Can you work these out from the model? Positions are in its coordinate system, mm. A direction names the side the tool comes from. Coordinates: 2 decimals unless noted, no trailing zeros. Loops run counter-clockwise (first coordinate to the right, second up) from the corner with the lowest first, then second, coordinate; pieces in that order, holes last.
```python
from build123d import *

# Parameters (mm, degrees)
SKETCH_2_R      = 5
EXTRUDE_1_DEPTH = 92
SKETCH_3_R      = 16
EXTRUDE_2_DEPTH = 25
SKETCH_4_R      = 16
SKETCH_4_R_2    = 11
EXTRUDE_3_DEPTH = 10
EXTRUDE_3_DRAFT = 5
FILLET_1_R      = 1


with BuildPart() as part:
    # 草图2 → 凸台-拉伸1 (new body)
    with BuildSketch(Plane(origin=(-136.095806698, 0, 0), x_dir=(0, 0, -1), z_dir=(1, 0, 0))):
        with Locations((-537.761833513, -181.314321461)):
            Circle(SKETCH_2_R)
    extrude(amount=-EXTRUDE_1_DEPTH)

    # 草图3 → 凸台-拉伸2 (add)
    with BuildSketch(Plane.ZY.offset(228.095806698)):
        with Locations((537.761833513, -181.314321461)):
            Circle(SKETCH_3_R)
    extrude(amount=EXTRUDE_2_DEPTH)


with BuildPart() as extrude_3_tool:
    # 草图4 → 凸台-拉伸3 (with draft: the straight prism first)
    with BuildSketch(Plane(origin=(-228.095806698, 0, 0), x_dir=(0, 0, -1), z_dir=(1, 0, 0))):
        with Locations((-537.761833513, -181.314321461)):
            Circle(SKETCH_4_R)
        with Locations((-537.761833513, -181.314321461)):
            Circle(SKETCH_4_R_2, mode=Mode.SUBTRACT)
    extrude(amount=EXTRUDE_3_DEPTH)
    # 凸台-拉伸3: the draft: its side faces are tilted about the plane it starts from
    extrude_3_sides = [extrude_3_tool.faces().sort_by_distance(p)[0] for p in [
        (-223.095806698, -181.314321461, 553.761833513),
        (-223.095806698, -181.314321461, 548.761833513),
    ]]
    draft(extrude_3_sides, Plane(origin=(-228.095806698, 0, 0), x_dir=(0, 0, -1), z_dir=(1, 0, 0)), EXTRUDE_3_DRAFT)


with BuildPart() as part_1:
    add(part.part)

    # 凸台-拉伸3: add extrude_3_tool
    add(extrude_3_tool.part)

    # 圆角1
    # the kernel refuses this fillet: 1 mm, written as the material it takes off along each edge
    with BuildSketch(Plane(origin=(-228.095806698, -181.314321461, 537.761833513), x_dir=(0, 0, 1), z_dir=(0, -1, 0))) as fillet_1_piece_1:
        with BuildLine():
            CenterArc((16 - FILLET_1_R, FILLET_1_R * 0.0436609429085), FILLET_1_R, 355, 5)
            Line((16 - FILLET_1_R * 0.0038053019083, -FILLET_1_R * 0.0434947998392), (16, 0))
            Line((16, 0), (16, FILLET_1_R * 0.0436609429085))
        make_face()
    revolve(axis=Axis((-228.095806698, -181.314321461, 537.761833513), (-1, 0, 0)), revolution_arc=180, mode=Mode.SUBTRACT)
    with BuildSketch(Plane(origin=(-228.095806698, -181.314321461, 537.761833513), x_dir=(0, 0, -1), z_dir=(0, 1, 0))) as fillet_1_piece_2:
        with BuildLine():
            CenterArc((16 - FILLET_1_R, FILLET_1_R * 0.0436609429085), FILLET_1_R, 355, 5)
            Line((16 - FILLET_1_R * 0.0038053019083, -FILLET_1_R * 0.0434947998392), (16, 0))
            Line((16, 0), (16, FILLET_1_R * 0.0436609429085))
        make_face()
    revolve(axis=Axis((-228.095806698, -181.314321461, 537.761833513), (-1, 0, 0)), revolution_arc=180, mode=Mode.SUBTRACT)


solid = part_1.part
```
Item 1: I'm going to push flat-ended pins straight in: P1, Ø6, axis at y = -192, z = 531.5, coming from the +X side; P2, Ø1.5, axis at y = -172.5, z = 539.5, coming from the +X side; P3, Ø5, axis at x = -214, y = -182, coming from the -Z side. Where does each tip first touch, or does it pass through?
Results are:
P1: stops at x = -218.1
P2: stops at x = -228.1
P3: stops at z = 532.76
Item 2: I need wall thicknesses on line 1 along Y through (x, z) = (-219, 538); line 2 along X through (y, z) = (-183.5, 527.5); line 3 along Y through (x, z) = (-196, 538). Which ranges of each line are inside material? Lowest first, please.
Results are:
line 1: y = -196.52 to -193.11, -186.31 to -176.32, -169.52 to -166.11
line 2: x = -253.1 to -228.1
line 3: y = -186.31 to -176.32
Item 3: Suppose I cut it at B-B, the plane x = -242.5. Please give me the cut outline in (y, z).
Results are:
outline: circle Ø32 at (-181.31, 537.76)
Item 4: On a 3-axis mill with a long thin cutter (end or side, diameter ignored), from which of +Z, -Z, +X, -X, +Y, -Y can I reach the whole of each face in a straight line? I mean faces 1 (the face through (-218.096, -188, 548)), 2 (the face through (-136.096, -181, 538)). Say none if no direction works.
Results are:
face 1: +X
face 2: +Z, -Z, +X, +Y, -Y
Item 5: Suppose I cut it at A-A, the plane x = -216. Please give me the cut outline in (y, z), plus the area to 3 significant figures.
Results are:
outline: circle Ø10 at (-181.31, 537.76)
area: 78.5 mm2
